```python
from build123d import *

# Parameters (mm, degrees)
F0_W     = 38.1
F0_H     = 41.91
F1_DEPTH = 5.08
F2_W     = 38.1
F2_H     = 5.08
F3_DEPTH = 63.5
F4_R     = 4.153748588
F5_DEPTH = 48.768
F6_R     = 12.7


with BuildPart() as f1:
    # F0 (on Top) → F1 (new body)
    with BuildSketch(Plane.XY):
        Rectangle(F0_W, F0_H)
    extrude(amount=F1_DEPTH)

    # F2 (on face) → F3 (join)
    with BuildSketch(Plane.XY.offset(5.08)):
        with Locations((0, 18.415)):
            Rectangle(F2_W, F2_H)
        with Locations((0, -18.415)):
            Rectangle(F2_W, F2_H)
    extrude(amount=F3_DEPTH)

    # F4 (on face) → F5 (cut)
    with BuildSketch(Plane.XZ.offset(20.955)):
        with Locations((0, 58.42)):
            Circle(F4_R)
    extrude(amount=-F5_DEPTH, mode=Mode.SUBTRACT)

    # F6
    f6_edges = [f1.edges().sort_by_distance(p)[0] for p in [
        (-19.05, -18.415, 68.58),
        (-19.05, 18.415, 68.58),
        (19.05, -18.415, 68.58),
        (19.05, 18.415, 68.58),
    ]]
    fillet(f6_edges, radius=F6_R)


solid = f1.part
```
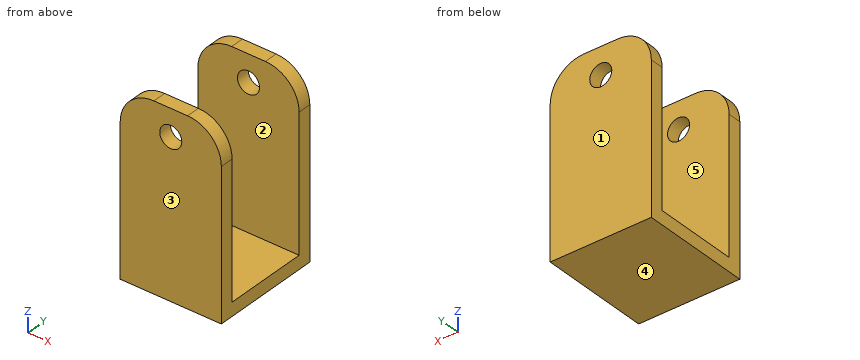
Design review of the part built by this model. Coordinates are the model's own, in mm. Face numbers are marked on the shaded views. A direction names the side the tool comes from. Give positions to 0.01 mm unless a question says otherwise; leave off trailing zeros. Write each loop counter-clockwise with the first axis right and the second up, starting at its lowest first coordinate (ties: lowest second). Pieces come first, ordered by that corner, then holes.
(1) Wall thickness on line 1 along Y through (x, z) = (5.5, 12) (3 decimals); line 2 along Z through (x, y) = (0, -19.35); line 3 along Z through (x, y) = (3.5, -4.5): over which ranges is each line inside the solid? List them lowest first.
Checked values:
line 1: y = -20.955 to -15.875, 15.875 to 20.955
line 2: z = 0 to 54.27, 62.57 to 68.58
line 3: z = 0 to 5.08
(2) Clearance check with a flat-ended pin moving along its axis: pin 1 Ø3 at (x, y) = (-7.5, 7.5) entering from +Z. State where the tip first meets the part, or that it passes through.
Checked values:
pin 1: stops at z = 5.08
(3) Mouldability with a two-part tool opening along Y and no side actions: class the marked faces 3, 4 and 5 as +Y half, -Y half, draft (parallel to the pull), parting line (faces both ways), or undercut.
Checked values:
face 3: -Y half
face 4: draft
face 5: undercut
(4) Add section C-C (z = 60.5). Give the boundary of the cut face in (x, y) (3 decimals), and give its area (3 significant figures).
Checked values:
outline: (-18.18, -20.955) - (-3.595, -20.955) - (-3.595, -15.875) - (-18.18, -15.875) - close; (-18.18, 15.875) - (-3.595, 15.875) - (-3.595, 20.955) - (-18.18, 20.955) - close; (3.595, -20.955) - (18.18, -20.955) - (18.18, -15.875) - (3.595, -15.875) - close; (3.595, 15.875) - (18.18, 15.875) - (18.18, 20.955) - (3.595, 20.955) - close
area: 296 mm2
(5) Add section B-B (z = 23.5). Give the boundary of the cut face in (x, y) (3 decimals).
Checked values:
outline: (-19.05, -20.955) - (19.05, -20.955) - (19.05, -15.875) - (-19.05, -15.875) - close; (-19.05, 15.875) - (19.05, 15.875) - (19.05, 20.955) - (-19.05, 20.955) - close
(6) Tool access review of the marked faces 1 and 2: name each direction out of +Z, -Z, +X, -X, +Y, -Y from which nothing blocks a thin tool from reaching the whole face with its end or side.
Checked values:
face 1: +Z, -Z, +X, -X, +Y
face 2: +Z, +X, -X
(7) Add section A-A (x = 0). Give the boundary of the cut face in (y, z) (3 decimals), and give its area (3 significant figures).
Checked values:
outline: (-20.955, 0) - (20.955, 0) - (20.955, 54.266) - (15.875, 54.266) - (15.875, 5.08) - (-15.875, 5.08) - (-15.875, 54.266) - (-20.955, 54.266) - close; (-20.955, 62.574) - (-15.875, 62.574) - (-15.875, 68.58) - (-20.955, 68.58) - close; (15.875, 62.574) - (20.955, 62.574) - (20.955, 68.58) - (15.875, 68.58) - close
area: 774 mm2
(8) Add section D-D (y = -5.5). Give the boundary of the cut face in (x, z).
Checked values:
outline: (-19.05, 0) - (19.05, 0) - (19.05, 5.08) - (-19.05, 5.08) - close
